from build123d import *

# Parameters (mm, degrees)
F1_DEPTH = 1625.6
F2_R     = 12.7


with BuildPart() as f1:
    # F0 (on Front) → F1 (new body)
    with BuildSketch(Plane.XZ):
        Polygon((6.35, -101.6), (101.6, -101.6), (101.6, -88.9), (6.35, -88.9), (6.35, 88.9), (101.6, 88.9), (101.6, 101.6), (-101.6, 101.6), (-101.6, 88.9), (-6.35, 88.9), (-6.35, -88.9), (-101.6, -88.9), (-101.6, -101.6), (-6.35, -101.6), align=None)
    extrude(amount=F1_DEPTH)

    # F2
    f2_edges = [f1.edges().sort_by_distance(p)[0] for p in [
        (-6.35, -812.8, -88.9),
        (6.35, -812.8, -88.9),
        (6.35, -812.8, 88.9),
        (-6.35, -812.8, 88.9),
    ]]
    fillet(f2_edges, radius=F2_R)


solid = f1.part
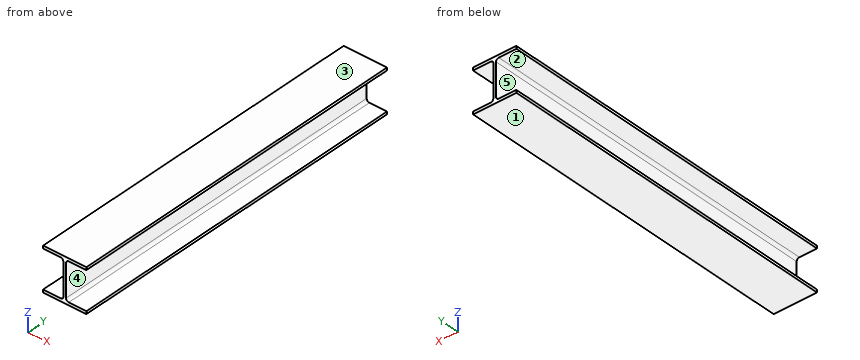
Part model, mm, in its own coordinate system. Face numbers are marked on the shaded views. A direction names the side the tool comes from. Coordinates: 2 decimals unless noted, no trailing zeros. Order: outer loops, then holes, each group sorted by start corner. A loop starts at its lowest first (then second) coordinate and runs counter-clockwise, first axis right, second up.
(1) Pull direction Z, two halves, no side cores. Call the marked faces 1, 2 and 3: pulls with the +Z half, pulls with the -Z half, needs draft (parallel to the pull), parting line crosses it, or undercut.
Check sheet entries:
face 1: pulls with the -Z half
face 2: undercut
face 3: pulls with the +Z half
(2) Slice it at A-A, the plane x = 87. Write the cut outline in (y, z).
Check sheet entries:
outline: (-1625.6, -101.6) - (0, -101.6) - (0, -88.9) - (-1625.6, -88.9) - close; (-1625.6, 88.9) - (0, 88.9) - (0, 101.6) - (-1625.6, 101.6) - close
(3) Slice it at B-B, the plane y = -943. Write the cut outline in (x, z), and give its area (3 significant figures).
Check sheet entries:
outline: (-101.6, -101.6) - (101.6, -101.6) - (101.6, -88.9) - (19.05, -88.9) arc R12.7 cw to (6.35, -76.2) - (6.35, 76.2) arc R12.7 cw to (19.05, 88.9) - (101.6, 88.9) - (101.6, 101.6) - (-101.6, 101.6) - (-101.6, 88.9) - (-19.05, 88.9) arc R12.7 cw to (-6.35, 76.2) - (-6.35, -76.2) arc R12.7 cw to (-19.05, -88.9) - (-101.6, -88.9) - close
area: 7,560 mm2
(4) Slice it at C-C, the plane z = 10.5. Write the cut outline in (x, y).
Check sheet entries:
outline: (-6.35, -1625.6) - (6.35, -1625.6) - (6.35, 0) - (-6.35, 0) - close
(5) Probe L1, parallel to Z at x = -87, y = -1089.5; L2, parallel to X at y = -1024.5, z = -67; L3, parallel to Z at x = -16.5, y = -289. List the from-to ranges inside material, lowest first.
Check sheet entries:
L1: z = -101.6 to -88.9, 88.9 to 101.6
L2: x = -6.35 to 6.35
L3: z = -101.6 to -88.64, 88.64 to 101.6
(6) Tool access for the marked faces 4 and 5: list every direction of +Z, -Z, +X, -X, +Y, -Y with a clear straight run to the whole face (end or side of a thin tool).
Check sheet entries:
face 4: +X, +Y, -Y
face 5: -X, +Y, -Y
